Can you work these out from the drawing? Everything is in mm from the part's minimum corner. A direction names the side the tool comes from. Round coordinates to 2 decimals unless told otherwise and drop trailing zeros. Order: outer loops, then holes, each group sorted by start corner. A loop starts at its lowest first (then second) coordinate and runs counter-clockwise, first axis right, second up. Notation, with made-up numbers: M 31,62.25 L 59,62.25 A4 cw 59,67.25 Z; hole C 70.25,-11.75 d5. An arc over 180 degrees is marked long. Write item = value, one per line. Start each with the question number.
Item 1: Please list where these lines run through material, in increasing order: L1, parallel to X at y = 0.75, z = 1.65; L2, parallel to Z at x = 1.5, y = 1.55; L3, parallel to Y at x = 0.75, z = 2.
Item 2: I want a section at A-A, the plane z = 1.5. List the corners of the cut face in (x, y) for me, plus the area to 4 significant figures.
Item 3: I want a section at C-C, the plane x = 10.25. List the corners of the cut face in (y, z) for me.
Item 4: I want a section at D-D, the plane y = 2.85. List the corners of the cut face in (x, z) for me.
Item 5: For the marked faces 1, 2 and 3, which set-ups out of +Z, -Z, +X, -X, +Y, -Y let a thin tool reach every point of the face, with its end or its side?
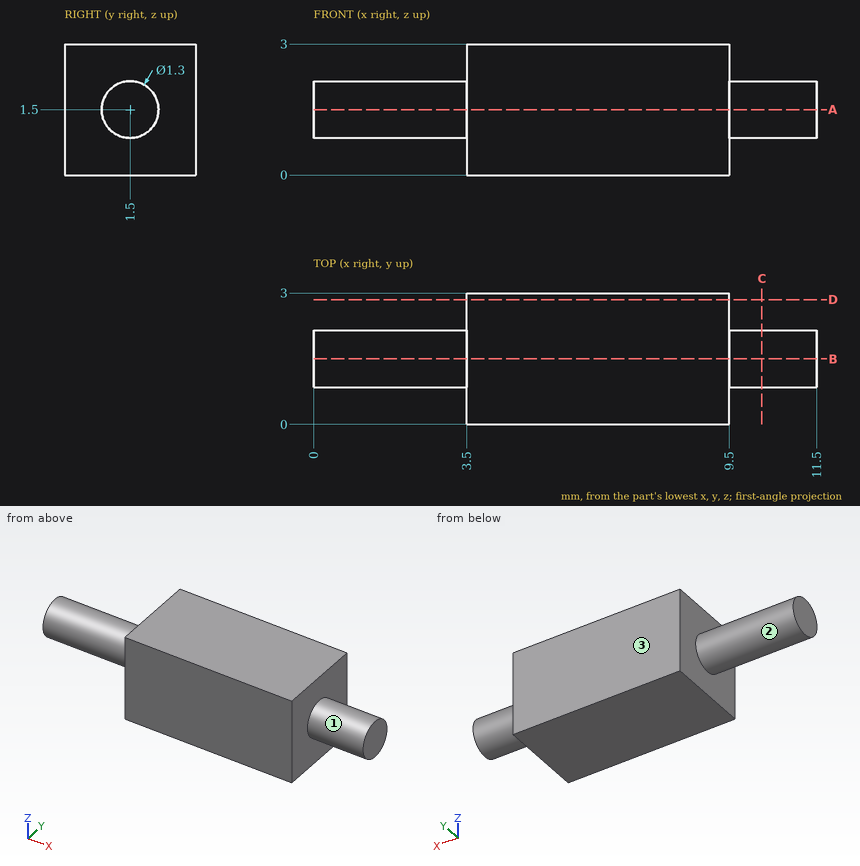
Filled in:
q1.L1 = 3.5 to 9.5
q1.L2 = 0.85 to 2.15
q1.L3 = 1.08 to 1.92
q2.outline = M 0,0.85 L 3.5,0.85 L 3.5,0 L 9.5,0 L 9.5,0.85 L 11.5,0.85 L 11.5,2.15 L 9.5,2.15 L 9.5,3 L 3.5,3 L 3.5,2.15 L 0,2.15 Z
q2.area = 25.15 mm^2
q3.outline = C 1.5,1.5 d1.3
q4.outline = M 3.5,0 L 9.5,0 L 9.5,3 L 3.5,3 Z
q5.face_1 = +X
q5.face_2 = -X
q5.face_3 = +Z, -Z, +X, -X, +Y
